Autodesk Inventor part; units mm, degrees
ref_plane "YZ Plane" through (0, 0, 0) normal (1, 0, 0) x (0, 1, 0)
ref_plane "XZ Plane" through (0, 0, 0) normal (0, 1, 0) x (-1, 0, 0)
ref_plane "XY Plane" through (0, 0, 0) normal (0, 0, 1) x (1, 0, 0)
sketch "Sketch1" plane through (0, 0, 0) normal (0, 1, 0) x (-1, 0, 0)
  line L0 (0, 0) -> (15, 0)
  line L1 (15, 0) -> (15, -34.5)
  line L2 (15, -34.5) -> (0, -34.5)
  line L3 (0, -34.5) -> (0, 0)
  line L4 (0, -17.25) -> (15, -17.25)
  circle A0 centre (7.5, -5.75) radius 1.675
  circle A1 centre (7.5, -28.75) radius 1.675
  circle A2 centre (-42.5, -5.75) radius 1.675
  line L5 (15, 0) -> (-50, 0)
  line L6 (-50, 0) -> (-50, -34.5)
  line L7 (-50, -34.5) -> (15, -34.5)
  line L8 (15, -34.5) -> (15, 0)
  circle A3 centre (-42.5, -28.75) radius 1.675
  point P0 (0, -34.5)
  dimension "d0" = 34.5
  dimension "d1" = 15
  dimension "d2" = 3.35
  dimension "d3" = 7.5
  dimension "d4" = 11.5
  dimension "d9" = 3.35
  dimension "d10" = 50
  dimension "d11" = 7.5
  dimension "d12" = 5.75
extrude "Plate1" add sketch "Sketch1" along normal blind 1.5
chamfer "Corner Chamfer1" distance 4 angle 45 4 edges at (-15, 0.75, 0) (-15, 0.75, -34.5) (50, 0.75, 0) (50, 0.75, -34.5)
equation "\"d0\" = 0.75 * A_width"
equation "\"d2\" = rivet_diameter"
equation "\"d3\" = 0.5 * d1"
equation "\"d4\" = 0.25 * A_width"
equation "\"d9\" = rivet_diameter"
equation "\"d5\" = Thickness"
equation "\"Thickness\" = thin_plate"
equation "\"BendRadius\" = Thickness"
equation "\"BendReliefWidth\" = Thickness"
equation "\"BendReliefDepth\" = 0.5 * Thickness"
equation "\"CornerReliefSize\" = 4 * Thickness"
equation "\"MinimumRemnant\" = 2 * Thickness"
equation "\"TransitionRadius\" = BendRadius"
equation "\"JacobiRadiusSize\" = BendRadius"
equation "\"GapSize\" = Thickness"
equation "\"A_width\" = 46"
equation "\"A_joint_diameter\" = 16"
equation "\"A_joint_tolerance\" = 3"
equation "\"l___________\" = 0"
equation "\"l__________\" = 0"
equation "\"l_________\" = 0"
equation "\"rivet_diameter\" = 3.35"
equation "\"plate_thickness\" = 3"
equation "\"l________\" = 0"
equation "\"A_B_spacing\" = 2"
equation "\"L_Piston_Bottom\" = 21"
equation "\"L_Piston_Top\" = 25"
equation "\"thin_plate\" = 1.5"
properties part number "A1_joiners" material "Stainless Steel"
Can you work these out from the model? Positions are in its coordinate system, mm. Coordinates: 2 decimals unless noted, no trailing zeros. Loops run counter-clockwise (first coordinate to the right, second up) from the corner with the lowest first, then second, coordinate; pieces in that order, holes last. Notation, with made-up numbers: (70, 73) - (120, 73) arc R20 cw to (120, 95) - close; hole circle Ø6 at (71, 69.25). An arc over 180 degrees is marked (long way). Answer as a JSON object with one key per item and string values. Group by question number.
Item 1: If I drill on L1, parallel to Z at x = 42.5, y = 0.6 (3 decimals); L2, parallel to X at y = 0.45, z = -30; L3, parallel to X at y = 0.8, z = -32, over which ranges is the centre line in solid material (lowest first)? Write a range as from..to.
Item 2: If we mould it in two halves opening along Z, with no side actions, what happens to faces 1 (the face through (-7.137, 0.74, -27.115)), 2 (the face through (18, 0, -17)), 3 (the face through (18, 1, -34.5))? For each: released by +Z, released by -Z, zero draft, split by the parting line, or undercut.
Item 3: If we section it at D-D (z = -2): List the corners of the cut face in (x, y) for me, plus the area to 3 significant figures.
Item 4: If we section it at C-C (y = 1.2): List the corners of the cut face in (x, z) for me (3 decimals), plus the area to 3 significant figures.
Item 5: If we section it at A-A (z = -5.75): List the corners of the cut face in (x, y) for me (3 decimals), plus the area to 4 significant figures.
Item 6: If we section it at B-B (x = 42.5): List the corners of the cut face in (y, z) for me (3 decimals).
Returned:
{
 "1": {"L1": "z = -34.5..-30.425, -27.075..-7.425, -4.075..0", "L2": "x = -15..-8.61, -6.39..41.39, 43.61..50", "L3": "x = -13.5..48.5"},
 "2": {"face 1": "undercut", "face 2": "zero draft", "face 3": "released by -Z"},
 "3": {"outline": "(-13, 0) - (48, 0) - (48, 1.5) - (-13, 1.5) - close", "area": "91.5 mm²"},
 "4": {"outline": "(-15, -30.5) - (-11, -34.5) - (46, -34.5) - (50, -30.5) - (50, -4) - (46, 0) - (-11, 0) - (-15, -4) - close; hole circle Ø3.35 at (-7.5, -28.75); hole circle Ø3.35 at (-7.5, -5.75); hole circle Ø3.35 at (42.5, -28.75); hole circle Ø3.35 at (42.5, -5.75)", "area": "2,180 mm²"},
 "5": {"outline": "(-15, 0) - (-9.175, 0) - (-9.175, 1.5) - (-15, 1.5) - close; (-5.825, 0) - (40.825, 0) - (40.825, 1.5) - (-5.825, 1.5) - close; (44.175, 0) - (50, 0) - (50, 1.5) - (44.175, 1.5) - close", "area": "87.45 mm²"},
 "6": {"outline": "(0, -34.5) - (1.5, -34.5) - (1.5, -30.425) - (0, -30.425) - close; (0, -27.075) - (1.5, -27.075) - (1.5, -7.425) - (0, -7.425) - close; (0, -4.075) - (1.5, -4.075) - (1.5, 0) - (0, 0) - close"}
}
